Part model, mm, in its own coordinate system. Face numbers are marked on the shaded views. A direction names the side the tool comes from. Round coordinates to 2 decimals unless told otherwise and drop trailing zeros. Loops run counter-clockwise (first coordinate to the right, second up) from the corner with the lowest first, then second, coordinate; pieces in that order, holes last. Notation, with made-up numbers: (76.5, 19) -> (86.5, 19) arc R10 ccw to (86.5, 36) -> close; hole circle Ø4 at (30, 44). An arc over 180 degrees is marked (long way). Use a Markdown table: item, result. Add a question column.
Item 1: Cut at B-B, the plane y = -3.5. List the corners of the cut face in (x, z).
Item 2: Flat gauge pins, fed straight in: pin 1 (12 mm diameter, centred on x = -8.5, z = 11, fed in from +Y); pin 2 (5 mm diameter, centred on y = -1.5, z = 11, fed in from -X); pin 3 (2 mm diameter, centred on x = -11.5, y = -4.5, fed in from +Z). Where does each tip first touch, or does it go through?
Item 3: Cut at C-C, the plane x = -14.25. List the corners of the cut face in (y, z), plus the area to 3 significant figures.
Item 4: Probe line 1 (Y direction, x = -14, z = 4.25); line 2 (Z direction, x = -5.25, y = -4.5). List the from-to ranges inside material, lowest first. Write a range as [from, to].
Item 5: Which spindle directions (+Z, -Z, +X, -X, +Y, -Y) get a long thin tool onto all of the face, cutting with end or side? Do the marked faces 4 and 5. Say none if no direction does.
Item 6: Cut at A-A, the plane z = 0.5. List the corners of the cut face in (x, y).
Item 7: Cut at D-D, the plane z = 9.75. List the corners of the cut face in (x, y).
Item 8: Two-plate mould, pull along Z, no slides. Class the marked faces 1, 2 and 3: pulls with the +Z half, pulls with the -Z half, needs draft (parallel to the pull), parting line crosses it, or undercut.
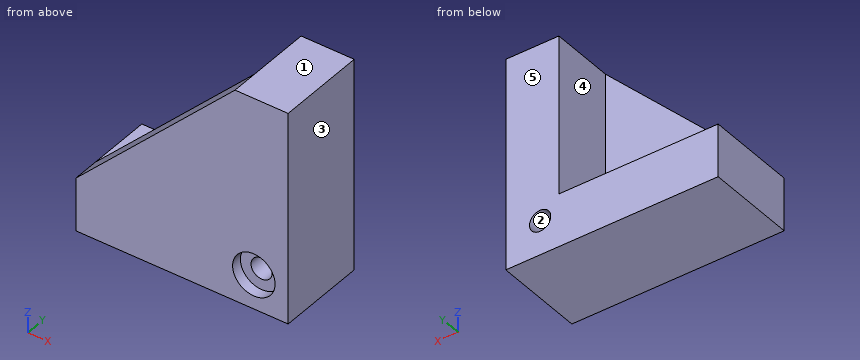
```python
from build123d import *

# Parameters (mm, degrees)
F1_DEPTH = 6
F3_DEPTH = 2.5
F4_R     = 1
F5_DEPTH = 8.501
F6_R     = 2
F7_DEPTH = 1


with BuildPart() as f1:
    # F0 (on Front) → F1 (new body)
    with BuildSketch(Plane.XZ):
        Polygon((3, -2), (3, 18), (-2, 18), (-2, 3), (-17, 3), (-17, -2), align=None)
    extrude(amount=F1_DEPTH)

    # F2 (on face) → F3 (join)
    with BuildSketch(Plane.XZ.offset(6)):
        Polygon((-2, 18), (-17, 3), (-17, -2), (3, -2), (3, 18), align=None)
    extrude(amount=F3_DEPTH)

    # F4 (on face) → F5 (cut, through all)
    with BuildSketch(Plane(origin=(0, 0, 0), x_dir=(-1, 0, 0), z_dir=(0, 1, 0))):
        with Locations((0.232233, 1.232233)):
            Circle(F4_R)
    extrude(amount=-F5_DEPTH, mode=Mode.SUBTRACT)

    # F6 (on face) → F7 (cut)
    with BuildSketch(Plane.XZ.offset(8.5)):
        with Locations((-0.232233, 1.232233)):
            Circle(F6_R)
    extrude(amount=-F7_DEPTH, mode=Mode.SUBTRACT)


solid = f1.part
```
A:
| question | item | result |
|---|---|---|
| 1 | outline | (-17, -2) -> (3, -2) -> (3, 18) -> (-2, 18) -> (-2, 3) -> (-17, 3) -> close; hole circle Ø2 at (-0.23, 1.23) |
| 2 | pin 1 | stops at y = -6 |
| 2 | pin 2 | stops at x = -2 |
| 2 | pin 3 | stops at z = 3 |
| 3 | outline | (-8.5, -2) -> (0, -2) -> (0, 3) -> (-6, 3) -> (-6, 5.75) -> (-8.5, 5.75) -> close |
| 3 | area | 49.4 mm^2 |
| 4 | line 1 | y = [-8.5, -6] |
| 4 | line 2 | z = [-2, 3] |
| 5 | face 4 | +Z, -X, +Y |
| 5 | face 5 | +Z, -Z, +X, -X, +Y |
| 6 | outline | (-17, -8.5) -> (-2.09, -8.5) -> (-2.09, -7.5) -> (-0.91, -7.5) -> (-0.91, 0) -> (-17, 0) -> close; (0.45, -7.5) -> (1.63, -7.5) -> (1.63, -8.5) -> (3, -8.5) -> (3, 0) -> (0.45, 0) -> close |
| 7 | outline | (-10.25, -8.5) -> (3, -8.5) -> (3, 0) -> (-2, 0) -> (-2, -6) -> (-10.25, -6) -> close |
| 8 | face 1 | pulls with the +Z half |
| 8 | face 2 | undercut |
| 8 | face 3 | needs draft |
